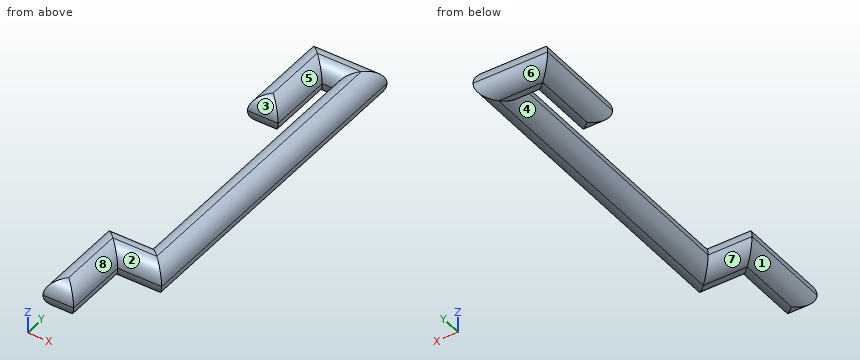
from build123d import *

# Parameters (mm, degrees)
EXTRU_MINCE1_DEPTH = 2.3
CONG_1_R           = 2.3


with BuildPart() as part:
    # Esquisse1 → Extru.-Mince1 (new, symmetric)
    with BuildSketch(Plane.XY):
        Polygon((-4.3, -57), (-4.3, -47.3), (2.3, -47.3), (2.3, 2.3), (-8.9, 2.3), (-8.9, -12), (-4.3, -12), (-4.3, -2.3), (-2.3, -2.3), (-2.3, -42.7), (-8.9, -42.7), (-8.9, -57), align=None)
    extrude(amount=EXTRU_MINCE1_DEPTH, both=True)

    # Congé1
    cong_1_edges = [part.edges().sort_by_distance(p)[0] for p in [
        (-6.6, -57, -2.3),
        (-4.3, -52.15, -2.3),
        (-1, -47.3, -2.3),
        (2.3, -22.5, -2.3),
        (-3.3, 2.3, -2.3),
        (-8.9, -4.85, -2.3),
        (-6.6, -12, -2.3),
        (-4.3, -7.15, -2.3),
        (-3.3, -2.3, -2.3),
        (-2.3, -22.5, -2.3),
        (-5.6, -42.7, -2.3),
        (-8.9, -49.85, -2.3),
        (-5.6, -42.7, 2.3),
        (-2.3, -22.5, 2.3),
        (-3.3, -2.3, 2.3),
        (-4.3, -7.15, 2.3),
        (-6.6, -12, 2.3),
        (-8.9, -4.85, 2.3),
        (-3.3, 2.3, 2.3),
        (2.3, -22.5, 2.3),
        (-1, -47.3, 2.3),
        (-4.3, -52.15, 2.3),
        (-6.6, -57, 2.3),
        (-8.9, -49.85, 2.3),
    ]]
    fillet(cong_1_edges, radius=CONG_1_R - 0.0001)  # a hair under: the kernel refuses the full size


solid = part.part
Input: part model. Units: mm. Frame: model coordinates. Face numbers are marked on the shaded views. A direction names the side the tool comes from. Give positions to 0.01 mm unless a question says otherwise; leave off trailing zeros. Order: outer loops, then holes, each group sorted by start corner. A loop starts at its lowest first (then second) coordinate and runs counter-clockwise, first axis right, second up. Notation, with made-up numbers: (64, 23.25) - (116, 23.25) arc R21 cw to (116, 60.25) - close; hole circle Ø6 at (77, 69.5). An arc over 180 degrees is marked (long way). Answer as a JSON object with one key per item and string values. Group by question number.
Q1. Cut plane D-D, the plane z = 1.6. Output: boundary loops of the cut face in (x, y).
Q2. Line query: probe 1 along Y at (x, z) = (-4.75, -1.5); probe 2 along Y at (x, z) = (-7.75, -0.4); probe 3 along Z at (x, y) = (-2, -20). Output: solid intervals per line, ascending.
Q3. First-contact query: pin 1 Ø1 at (x, z) = (-3.5, 0) entering from -Y; pin 2 Ø1.5 at (y, z) = (-16, -1.5) entering from +X. Flat tips, straight axial feed; report the tip coordinate or a pass-through.
Q4. Mould query, pull axis Y, two halves, no side actions, for the marked faces 6, 7 and 8. Classes: pulls with the +Y half, pulls with the -Y half, needs draft (parallel to the pull), parting line crosses it, or undercut.
Q5. Set-up query: the marked faces 1, 2, 3, 4 and 5. Return all of +Z, -Z, +X, -X, +Y, -Y with unobstructed straight access to the full face (end or side cutting, diameter ignored); none if empty.
Results:
{
 "1": {"outline": "(-8.25, -56.35) - (-4.95, -56.35) - (-4.95, -46.65) - (1.65, -46.65) - (1.65, 1.65) - (-8.25, 1.65) - (-8.25, -11.35) - (-4.95, -11.35) - (-4.95, -1.65) - (-1.65, -1.65) - (-1.65, -43.35) - (-8.25, -43.35) - close"},
 "2": {"probe 1": "-46.74 to -43.26, -1.74 to 1.74", "probe 2": "-56.96 to -42.74, -11.96 to 2.26", "probe 3": "-1.14 to 1.14"},
 "3": {"pin 1": "y = -47.3", "pin 2": "x = 2.17"},
 "4": {"face 6": "pulls with the +Y half", "face 7": "undercut", "face 8": "needs draft"},
 "5": {"face 1": "-Z, -X, +Y, -Y", "face 2": "+Z, +X, -Y", "face 3": "+Z, -X", "face 4": "-Z", "face 5": "+Z"}
}
